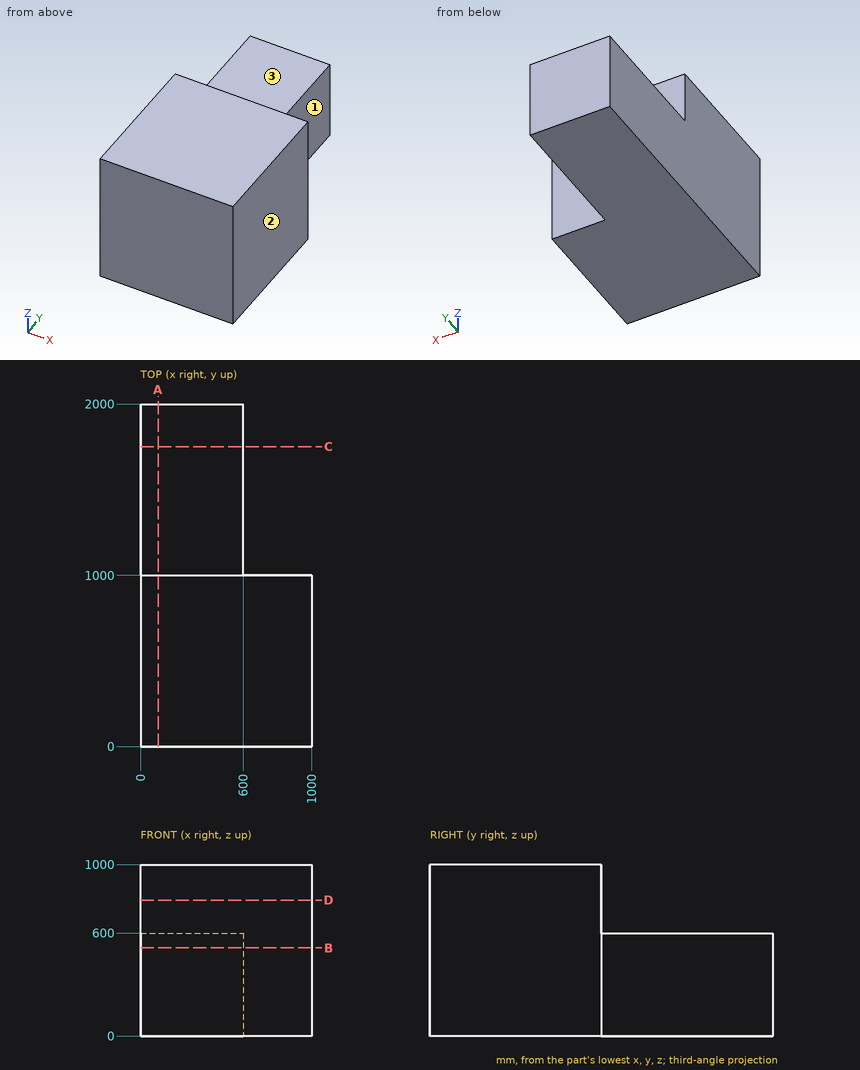
Check sheet for the drawn part. Datum: minimum x, y, z corner. Units: mm. A direction names the side the tool comes from. Round coordinates to 2 decimals unless told otherwise and drop trailing zeros. Write each loop counter-clockwise with the first axis right and the second up, starting at its lowest first coordinate (ties: lowest second). Pieces come first, ordered by that corner, then holes. Notation, with made-up numbers: (-1.5, -9.75) -> (49.5, -9.75) arc R15 ccw to (49.5, 9.25) -> close; hole circle Ø11 at (80, 32). An arc over 180 degrees is marked (long way). One line per item, written item: value. Start each with the question number.
(1) Scan lines: line 1 (Y direction, x = 304, z = 604); line 2 (X direction, y = 1105, z = 586.5). Record each from-to range of solid material in increasing order. Write a range as [from, to].
(2) Cross-section at C-C, the plane y = 1751. Record the cut outline in (x, z), and give its area (3 significant figures).
(3) Cross-section at D-D, the plane z = 793. Record the cut outline in (x, y).
(4) Cross-section at B-B, the plane z = 515. Record the cut outline in (x, y).
(5) Cross-section at A-A, the plane x = 103. Record the cut outline in (y, z), and give its area (3 significant figures).
(6) Access from +Z, -Z, +X, -X, +Y, -Y to the whole of each face (thin tool, end or side, straight path). Record for the marked faces 1, 2 and 3.
(7) Go/stop test with flat-tipped pins: pin 1 Ø4 at (y, z) = (426, 720) entering from -X; pin 2 Ø1 at (x, y) = (329.5, 1626) entering from +Z; pin 3 Ø1.5 at (x, z) = (371.5, 794) entering from +Y; pin 4 Ø5 at (y, z) = (1409, 557) entering from +X. Record where each tip stops, or that it passes through.
Answer:
1. line 1: [0, 1000]
1. line 2: [0, 600]
2. outline: (0, 0) -> (600, 0) -> (600, 600) -> (0, 600) -> close
2. area: 360,000 mm²
3. outline: (0, 0) -> (1000, 0) -> (1000, 1000) -> (0, 1000) -> close
4. outline: (0, 0) -> (1000, 0) -> (1000, 1000) -> (600, 1000) -> (600, 2000) -> (0, 2000) -> close
5. outline: (0, 0) -> (2000, 0) -> (2000, 600) -> (1000, 600) -> (1000, 1000) -> (0, 1000) -> close
5. area: 1,600,000 mm²
6. face 1: +Z, -Z, +X, +Y
6. face 2: +Z, -Z, +X, +Y, -Y
6. face 3: +Z, +X, -X, +Y
7. pin 1: x = 0
7. pin 2: z = 600
7. pin 3: y = 1000
7. pin 4: x = 600
